Check sheet for the drawn part. Datum: minimum x, y, z corner. Units: mm. Round coordinates to 2 decimals unless told otherwise and drop trailing zeros. Write each loop counter-clockwise with the first axis right and the second up, starting at its lowest first coordinate (ties: lowest second). Pieces come first, ordered by that corner, then holes. Notation, with made-up numbers: (55, 2) - (68, 2) arc R7 ccw to (68, 13) - close; hole circle Ø2 at (17.5, 1). An arc over 180 degrees is marked (long way). Answer as a JSON object with one key per item and string values.
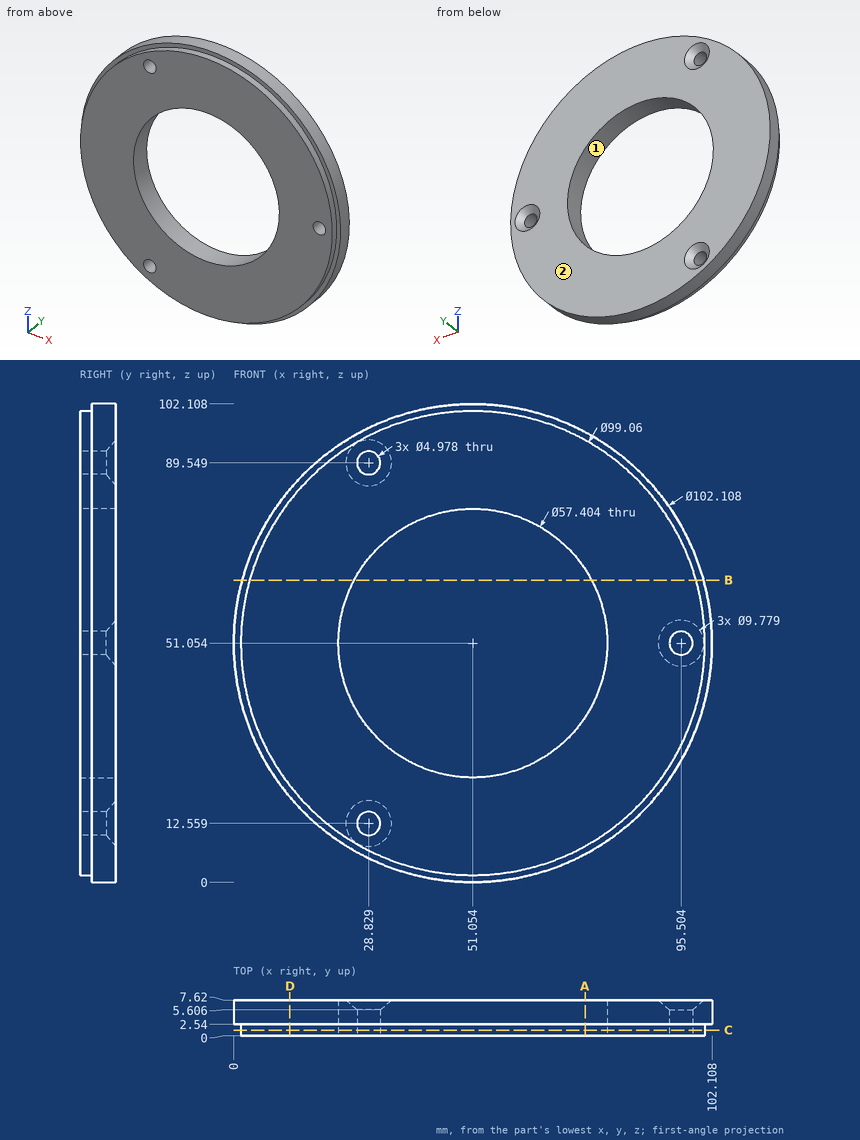
1. Cross-section at A-A (x = 75). Record the boundary of the cut face in (y, z), plus the area to 3 significant figures.
Completed:
{"outline": "(0, 7.7) - (2.54, 7.7) - (2.54, 5.96) - (7.62, 5.96) - (7.62, 35.23) - (0, 35.23) - close; (0, 66.88) - (7.62, 66.88) - (7.62, 96.14) - (2.54, 96.14) - (2.54, 94.41) - (0, 94.41) - close", "area": "437 mm^2"}
2. Cross-section at D-D (x = 12). Record the boundary of the cut face in (y, z).
Completed:
{"outline": "(0, 20.59) - (2.54, 20.59) - (2.54, 18.17) - (7.62, 18.17) - (7.62, 83.94) - (2.54, 83.94) - (2.54, 81.52) - (0, 81.52) - close"}
3. Cross-section at C-C (y = 1.25). Record the boundary of the cut face in (x, z) (1 decimal).
Completed:
{"outline": "circle Ø99.1 at (51.1, 51.1); hole circle Ø57.4 at (51.1, 51.1); hole circle Ø5 at (28.8, 12.6); hole circle Ø5 at (28.8, 89.5); hole circle Ø5 at (95.5, 51.1)"}
4. Material ranges on probe 1 along Z at (x, y) = (44, 3.5) (1 decimal); probe 2 along Z at (x, y) = (41.5, 3.25) (1 decimal); probe 3 along X at (y, z) = (4.25, 39) (1 decimal), recorded low to high. Write a range as from..to.
Completed:
{"probe 1": "z = 0.5..23.2, 78.9..101.6", "probe 2": "z = 0.9..24, 78.1..101.2", "probe 3": "x = 1.4..25, 77.1..100.7"}
5. Cross-section at B-B (z = 64.5). Record the boundary of the cut face in (x, y) (1 decimal), plus the area to 3 significant figures.
Completed:
{"outline": "(1.8, 2.5) - (3.4, 2.5) - (3.4, 0) - (25.7, 0) - (25.7, 7.6) - (1.8, 7.6) - close; (76.4, 0) - (98.7, 0) - (98.7, 2.5) - (100.3, 2.5) - (100.3, 7.6) - (76.4, 7.6) - close", "area": "356 mm^2"}
6. Go/stop test with flat-tipped pins: pin 1 (3 mm diameter, centred on x = 23, y = 1, fed in from +Z) (1 decimal); pin 2 (3 mm diameter, centred on x = 28.83, z = 89.55, fed in from +Y); pin 3 (2 mm diameter, centred on y = 4, z = 15.5, fed in from -X); pin 4 (5.5 mm diameter, centred on x = 95.504, z = 51.054, fed in from -Y). Record where each tip stops, or that it passes through.
Completed:
{"pin 1": "stops at z = 92.9", "pin 2": "passes through", "pin 3": "stops at x = 13.47", "pin 4": "stops at y = 0"}
7. Mould release check, pull along X, two halves, no side actions. Record for the marked faces 1 and 2: released by +X, released by -X, zero draft, split by the parting line, or undercut.
Completed:
{"face 1": "undercut", "face 2": "zero draft"}
